from build123d import *

# Parameters (mm, degrees)
SKETCH_W        = 54.4
SKETCH_H        = 115
PAD_DEPTH       = 92
SKETCH001_W     = 50.4
SKETCH001_H     = 111
POCKET_DEPTH    = 90
POCKET001_DEPTH = 3
SKETCH003_R     = 1.7
POCKET002_DEPTH = 3
POCKET003_DEPTH = 18.99
POCKET004_DEPTH = 2.02
SKETCH006_R     = 5
SKETCH006_R_2   = 1.7
PAD001_DEPTH    = 1.6
POCKET005_DEPTH = 1.8
SKETCH008_R     = 7
PAD002_DEPTH    = 1
PAD003_DEPTH    = 8
POCKET006_DEPTH = 1.5
SKETCH011_R     = 2.8
POCKET007_DEPTH = 54.401
SKETCH012_R     = 7
PAD004_DEPTH    = 1
SKETCH013_R     = 2.8
POCKET008_DEPTH = 4
CHAMFER_SIZE    = 0.98
CHAMFER001_SIZE = 1.58


with BuildPart() as part:
    # Sketch → Pad (new body)
    with BuildSketch(Plane.XY):
        with Locations((27.2, 57.5)):
            Rectangle(SKETCH_W, SKETCH_H)
    extrude(amount=PAD_DEPTH)

    # Sketch001 → Pocket (cut)
    with BuildSketch(Plane.XY.offset(92)):
        with Locations((27.2, 57.5)):
            Rectangle(SKETCH001_W, SKETCH001_H)
    extrude(amount=-POCKET_DEPTH, mode=Mode.SUBTRACT)

    # Sketch002 → Pocket001 (cut)
    with BuildSketch(Plane.XZ):
        with BuildLine():
            Line((3, 23), (44, 23))
            ThreePointArc((44, 17), (47, 20), (44, 23))
            Line((44, 17), (3, 17))
            Line((3, 17), (3, 23))
        make_face()
    extrude(amount=-POCKET001_DEPTH, mode=Mode.SUBTRACT)

    # Sketch003 → Pocket002 (cut)
    with BuildSketch(Plane.XZ.offset(-115)):
        with Locations((7.2, 38)):
            Circle(SKETCH003_R)
        with Locations((47.2, 38)):
            Circle(SKETCH003_R)
        Polygon((13.3, 61.9), (41.1, 61.9), (41.1, 19.85), (35.35, 14.1), (19.05, 14.1), (13.3, 19.85), align=None)
    extrude(amount=POCKET002_DEPTH, mode=Mode.SUBTRACT)

    # Sketch004 → Pocket003 (cut, symmetric)
    with BuildSketch(Plane.XY.offset(21)):
        Polygon((0, 0), (18.8, 0), (18.8, 2.4), (2.4, 18.8), (0, 18.8), align=None)
    extrude(amount=POCKET003_DEPTH, both=True, mode=Mode.SUBTRACT)

    # Sketch005 → Pocket004 (cut)
    with BuildSketch(Plane.YZ):
        with BuildLine():
            Line((106, 29.757359), (106, 19))
            ThreePointArc((101, 14), (104.535534, 15.464466), (106, 19))
            Line((101, 14), (93, 14))
            ThreePointArc((88, 19), (89.464466, 15.464466), (93, 14))
            Line((88, 19), (88, 29.757359))
            ThreePointArc((89.464466, 33.292893), (88.380602, 31.670776), (88, 29.757359))
            Line((89.464466, 33.292893), (95.585786, 39.414214))
            ThreePointArc((98.414214, 39.414214), (97, 40), (95.585786, 39.414214))
            Line((98.414214, 39.414214), (104.535534, 33.292893))
            ThreePointArc((106, 29.757359), (105.619398, 31.670777), (104.535534, 33.292893))
        make_face()
    extrude(amount=POCKET004_DEPTH, mode=Mode.SUBTRACT)

    # Sketch006 → Pad001 (join)
    with BuildSketch(Plane.XZ.offset(-113)):
        with Locations((7.2, 38)):
            Circle(SKETCH006_R)
        with Locations((7.2, 38)):
            Circle(SKETCH006_R_2, mode=Mode.SUBTRACT)
        with Locations((47.2, 38)):
            Circle(SKETCH006_R)
        with Locations((47.2, 38)):
            Circle(SKETCH006_R_2, mode=Mode.SUBTRACT)
    extrude(amount=PAD001_DEPTH)

    # Sketch007 → Pocket005 (cut)
    with BuildSketch(Plane.XZ.offset(-111.4)):
        Polygon((7.2, 41.290897), (4.35, 39.645448), (4.35, 36.354552), (7.2, 34.709103), (10.05, 36.354552), (10.05, 39.645448), align=None)
        Polygon((47.2, 41.290897), (44.35, 39.645448), (44.35, 36.354552), (47.2, 34.709103), (50.05, 36.354552), (50.05, 39.645448), align=None)
    extrude(amount=-POCKET005_DEPTH, mode=Mode.SUBTRACT)

    # Sketch008 → Pad002 (join)
    with BuildSketch(Plane.YZ.offset(2)):
        with Locations((28, 30)):
            Circle(SKETCH008_R)
        with Locations((74, 30)):
            Circle(SKETCH008_R)
        with Locations((74, 10)):
            Circle(SKETCH008_R)
    extrude(amount=PAD002_DEPTH)

    # Sketch009 → Pad003 (join)
    with BuildSketch(Plane.YZ.offset(52.4)):
        with BuildLine():
            Line((31.535537, 26.46447), (29, 23.928932))
            Line((29, 23.928932), (29, 15.928932))
            Line((29, 15.928932), (27, 15.928932))
            Line((27, 15.928932), (27, 23.928932))
            Line((27, 23.928932), (24.464463, 26.46447))
            ThreePointArc((31.535537, 26.46447), (28, 35), (24.464463, 26.46447))
        make_face()
        with BuildLine():
            Line((77.535537, 26.46447), (75, 23.928932))
            Line((75, 23.928932), (75, 16.071068))
            Line((77.535528, 13.53554), (75, 16.071068))
            ThreePointArc((77.535519, 6.464451), (79, 9.999994), (77.535528, 13.53554))
            Line((77.535519, 6.464451), (74.999974, 3.928932))
            Line((74.999974, 1), (74.999974, 3.928932))
            Line((72.999974, 1), (74.999974, 1))
            Line((72.999974, 3.928932), (72.999974, 1))
            Line((70.464455, 6.464477), (72.999974, 3.928932))
            ThreePointArc((70.464461, 13.535528), (69, 10.000004), (70.464455, 6.464477))
            Line((70.464461, 13.535528), (73, 16.071068))
            Line((73, 16.071068), (73, 23.928932))
            Line((73, 23.928932), (70.464463, 26.46447))
            ThreePointArc((77.535537, 26.46447), (74, 35), (70.464463, 26.46447))
        make_face()
    extrude(amount=-PAD003_DEPTH)

    # Sketch010 → Pocket006 (cut, symmetric)
    with BuildSketch(Plane.XZ.offset(-28)):
        Polygon((44.4, 23.928932), (52.4, 15.928932), (44.4, 15.928932), align=None)
    extrude(amount=POCKET006_DEPTH, both=True, mode=Mode.SUBTRACT)

    # Sketch011 → Pocket007 (cut, through all)
    with BuildSketch(Plane.YZ):
        with Locations((28, 30)):
            Circle(SKETCH011_R)
        with Locations((74, 30)):
            Circle(SKETCH011_R)
        with Locations((74, 10)):
            Circle(SKETCH011_R)
    extrude(amount=POCKET007_DEPTH, mode=Mode.SUBTRACT)

    # Sketch012 → Pad004 (join)
    with BuildSketch(Plane.XZ.offset(-2)):
        with Locations((30, 74)):
            Circle(SKETCH012_R)
    extrude(amount=-PAD004_DEPTH)

    # Sketch013 → Pocket008 (cut)
    with BuildSketch(Plane.XZ):
        with Locations((30, 74)):
            Circle(SKETCH013_R)
    extrude(amount=-POCKET008_DEPTH, mode=Mode.SUBTRACT)

    # Chamfer
    chamfer_edges = [part.edges().sort_by_distance(p)[0] for p in [
        (3, 21, 30),
        (3, 67, 30),
        (3, 67, 10),
    ]]
    chamfer(chamfer_edges, length=CHAMFER_SIZE)

    # Chamfer001
    chamfer001_edges = [part.edges().sort_by_distance(p)[0] for p in [
        (42.2, 111.4, 38),
        (2.2, 111.4, 38),
    ]]
    chamfer(chamfer001_edges, length=CHAMFER001_SIZE)


solid = part.part
Work out the finished part from the listing and answer in its coordinate system (mm). A direction names the side the tool comes from. Give positions to 0.01 mm unless a question says otherwise; leave off trailing zeros. Order: outer loops, then holes, each group sorted by start corner. A loop starts at its lowest first (then second) coordinate and runs counter-clockwise, first axis right, second up. Notation, with made-up numbers: (38, -36.75) - (43, -36.75) arc R11 ccw to (43, -18.75) - close; hole circle Ø3 at (54.5, -20). An arc over 180 degrees is marked (long way). Answer as CSV lines item,"result". Start each with the question number.
Q1. The part is cut by section D-D (z = 64). Write down the section's boundary in (x, y), then the cut area to 3 significant figures.
Q2. The part is cut by section A-A (x = 30). Write down the section's boundary in (y, z).
Q3. Find the intervals of material crossed by L1, parallel to X at y = 114.1, z = 38; L2, parallel to Z at x = 30, y = 2.4; L3, parallel to Y at x = 47, z = 30, in increasing order. Write a range as [from, to].
Q4. The mould has two halves that part along X. Classify faces 5 (the face through (29.09, 2.49, 80.94)), 6 (the face through (48.456, 71.714, 14.786)), 7 (the face through (49.33, 76.67, 30.84)): +X half, -X half, draft (parallel to the pull), parting line (faces both ways), or undercut.
Q5. For faces 1 (the face through (1, 89, 16)), 2 (the face through (48.46, 71.75, 25.18)), 3 (the face through (30, 3, 71)), 4 (the face through (3, 75, 7)), determine the directions among +Z, -Z, +X, -X, +Y, -Y from which every point of the face is accessible in a straight line to the end or side of a thin tool.
Q6. The part is cut by section C-C (x = 39). Write down the section's boundary in (y, z), then the cut area to 3 significant figures.
Q7. Given pin 1 Ø4.5 at (x, z) = (30, 74) entering from -Y; pin 2 Ø10 at (x, z) = (28, 20) entering from +Y; pin 3 Ø3 at (x, y) = (24, 41.5) entering from +Z, each flat-ended and moving along its own axis, determine where each tip first touches the part or whether it passes through.
Check result:
1,outline,"(0, 0) - (54.4, 0) - (54.4, 115) - (0, 115) - close; hole (2, 2) - (52.4, 2) - (52.4, 113) - (2, 113) - close"
1,area,"662 mm²"
2,outline,"(0, 0) - (115, 0) - (115, 14.1) - (113, 14.1) - (113, 2) - (2, 2) - (2, 17) - (0, 17) - close; (0, 23) - (2, 23) - (2, 67) - (3, 67) - (3, 71.2) - (0, 71.2) - close; (0, 76.8) - (3, 76.8) - (3, 81) - (2, 81) - (2, 92) - (0, 92) - close; (113, 61.9) - (115, 61.9) - (115, 92) - (113, 92) - close"
3,L1,"x = [0, 5.5], [8.9, 13.3], [41.1, 45.5], [48.9, 54.4]"
3,L2,"z = [0, 2], [67, 71.2], [76.8, 81]"
3,L3,"y = [0, 2], [23, 25.2], [30.8, 33], [69, 71.2], [76.8, 79], [113, 115]"
4,face 5,"undercut"
4,face 6,"undercut"
4,face 7,"draft"
5,face 1,"-X"
5,face 2,"none"
5,face 3,"+Z"
5,face 4,"+Z, -Y"
6,outline,"(0, 0) - (115, 0) - (115, 17.75) - (113, 17.75) - (113, 2) - (2, 2) - (2, 17) - (0, 17) - close; (0, 23) - (2, 23) - (2, 92) - (0, 92) - close; (113, 61.9) - (115, 61.9) - (115, 92) - (113, 92) - close"
6,area,"490 mm²"
7,pin 1,"stops at y = 113"
7,pin 2,"stops at y = 2"
7,pin 3,"stops at z = 2"
